Input: part model. Units: mm. Frame: model coordinates. Face numbers are marked on the shaded views. A direction names the side the tool comes from. Give positions to 0.01 mm unless a question says otherwise; leave off trailing zeros. Write each loop counter-clockwise with the first axis right and the second up, starting at its lowest first coordinate (ties: lowest second). Pieces come first, ordered by that corner, then holes.
```python
from build123d import *

# Parameters (mm, degrees)
F1_DEPTH = 38.1
F2_R     = 11.430216
F3_DEPTH = 16.495738
F4_R     = 15.667724
F4_R_2   = 11.430216
F5_DEPTH = 6.858
F7_DEPTH = 13.431763


with BuildPart() as f1:
    # F0 (on Front) → F1 (new body, symmetric)
    with BuildSketch(Plane.XZ):
        Polygon((-49.148042, 0), (0, 0), (0, 75.40103), (-16.495738, 75.40103), (-16.495738, 13.431763), (-49.148042, 13.431763), align=None)
    extrude(amount=F1_DEPTH, both=True)

    # F2 (on face) → F3 (cut, through all)
    with BuildSketch(Plane(origin=(-16.495738, 0, 0), x_dir=(0, -1, 0), z_dir=(-1, 0, 0))):
        with Locations((0, 56.321822)):
            Circle(F2_R)
    extrude(amount=-F3_DEPTH, mode=Mode.SUBTRACT)

    # F4 (on face) → F5 (cut)
    with BuildSketch(Plane(origin=(-16.495738, 0, 0), x_dir=(0, -1, 0), z_dir=(-1, 0, 0))):
        with Locations((0, 56.321822)):
            Circle(F4_R)
        with Locations((0, 56.321822)):
            Circle(F4_R_2, mode=Mode.SUBTRACT)
    extrude(amount=-F5_DEPTH, mode=Mode.SUBTRACT)

    # F6 (on face) → F7 (cut, through all)
    with BuildSketch(Plane.XY.offset(13.431763)):
        with BuildLine():
            ThreePointArc((-37.367893, -9.263817), (-30.573506, -6.685717), (-27.725438, 0))
            ThreePointArc((-27.725438, 0), (-30.374154, 6.488307), (-36.806871, 9.269308))
            Line((-36.806871, 9.269308), (-37.186506, 9.269308))
            ThreePointArc((-37.186506, 9.269308), (-46.267496, 0.090735), (-37.367893, -9.263817))
        make_face()
        with BuildLine():
            Line((-49.148042, -9.263817), (-37.367893, -9.263817))
            ThreePointArc((-37.367893, -9.263817), (-46.267496, 0.090735), (-37.186506, 9.269308))
            Line((-37.186506, 9.269308), (-49.148042, 9.269308))
            Line((-49.148042, 9.269308), (-49.148042, -9.263817))
        make_face()
    extrude(amount=-F7_DEPTH, mode=Mode.SUBTRACT)


solid = f1.part
```
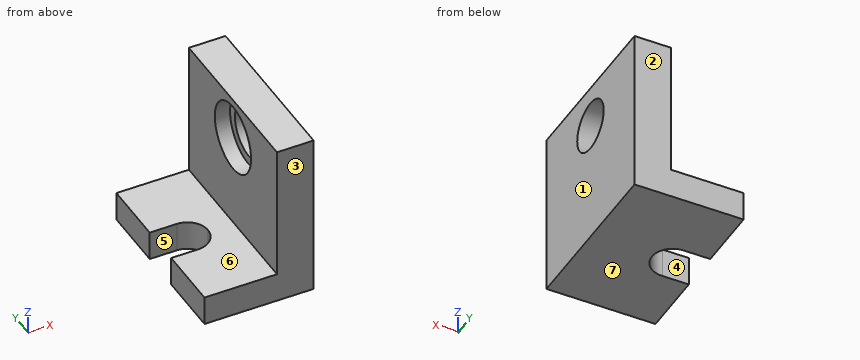
Item 1: Mould query, pull axis Y, two halves, no side actions, for the marked faces 1, 2, 3 and 4. Classes: +Y half, -Y half, draft (parallel to the pull), parting line (faces both ways), or undercut.
Item 2: Ray query, line 1 (Z direction, x = -3, y = 0); line 2 (Y direction, x = -42, z = 11); line 3 (Z direction, x = -18, y = 1). Return the intervals inside material, ascending.
Item 3: Pin query (flat end, axial travel): pin 1 (4 mm diameter, centred on x = -8, y = 13, fed in from -Z); pin 2 (13.5 mm diameter, centred on y = 0, z = 56.32, fed in from -X) (3 decimals); pin 3 (10 mm diameter, centred on x = -32.5, y = 22, fed in from +Z); pin 4 (15.5 mm diameter, centred on y = 3.5, z = 49, fed in from -X). Return the tip coordinate at first contact, or that it passes through.
Item 4: Section B-B (y = 1.5). Return loops of the section in (x, z), and give its area (3 significant figures).
Item 5: Section D-D (z = 43.5). Return loops of the section in (x, y).
Item 6: Section A-A (x = -45.5). Return loops of the section in (y, z).
Item 7: Section C-C (z = 62). Return loops of the section in (x, y), and give its area (3 significant figures).
Item 8: Set-up query: the marked faces 5, 6 and 7. Return all of +Z, -Z, +X, -X, +Y, -Y with unobstructed straight access to the full face (end or side cutting, diameter ignored); none if empty.
Solved:
1. face 1: draft
1. face 2: +Y half
1. face 3: -Y half
1. face 4: undercut
2. line 1: z = 0 to 44.89, 67.75 to 75.4
2. line 2: y = -38.1 to -9.26, 9.27 to 38.1
2. line 3: z = 0 to 13.43
3. pin 1: stops at z = 0
3. pin 2: passes through
3. pin 3: stops at z = 13.43
3. pin 4: stops at x = -16.5
4. outline: (-27.85, 0) - (0, 0) - (0, 44.99) - (-9.64, 44.99) - (-9.64, 40.73) - (-16.5, 40.73) - (-16.5, 13.43) - (-27.85, 13.43) - close; (-16.5, 71.92) - (-9.64, 71.92) - (-9.64, 67.65) - (0, 67.65) - (0, 75.4) - (-16.5, 75.4) - close
4. area: 964 mm2
5. outline: (-16.5, -38.1) - (0, -38.1) - (0, 38.1) - (-16.5, 38.1) - (-16.5, 9) - (-9.64, 9) - (-9.64, -9) - (-16.5, -9) - close
6. outline: (-38.1, 0) - (-9.26, 0) - (-9.26, 13.43) - (-38.1, 13.43) - close; (9.27, 0) - (38.1, 0) - (38.1, 13.43) - (9.27, 13.43) - close
7. outline: (-16.5, -38.1) - (0, -38.1) - (0, -9.92) - (-9.64, -9.92) - (-9.64, -14.6) - (-16.5, -14.6) - close; (-16.5, 14.6) - (-9.64, 14.6) - (-9.64, 9.92) - (0, 9.92) - (0, 38.1) - (-16.5, 38.1) - close
7. area: 865 mm2
8. face 5: +Z, -Z, -X
8. face 6: +Z, -X, +Y, -Y
8. face 7: -Z, +X, -X, +Y, -Y
